The figure shows three views and two pictorial views of one solid part (mm, origin at its lowest corner). Answer the questions. A direction names the side the tool comes from. Give positions to 0.01 mm unless a question says otherwise; leave off trailing zeros. Order: outer loops, then holes, each group sorted by start corner. A loop starts at its lowest first (then second) coordinate and runs counter-clockwise, first axis right, second up. Notation, with made-up numbers: (86.25, -8.5) - (138.25, -8.5) arc R25 cw to (138.25, 13.5) - close; hole circle Ø6 at (35.25, -26). An arc over 180 degrees is marked (long way). Use a Markdown table: item, result. Add a question column.
1. A cutting plane is placed at A-A on y = 2.1. Determine the outline of the cut face in (x, z).
2. A cutting plane is placed at B-B on x = 2. Determine the outline of the cut face in (y, z), and give its area (3 significant figures).
3. For a pull along X with two mould halves and no side action, classify the marked faces 3, 4 and 5 as released by +X, released by -X, zero draft, split by the parting line, or undercut.
4. Consider L1, parallel to X at y = 6.25, z = 4.8 (3 decimals); L2, parallel to Y at x = 2.5, z = 3; L3, parallel to Y at x = 2.5, z = 5.25. Determine where each line is inside the solid, lowest interval first.
5. Which of the six approach directions +Z, -Z, +X, -X, +Y, -Y give full straight-line access (tool end or side, diameter ignored) to the marked faces 1 and 2?
6. A cutting plane is placed at D-D on y = 8.75. Determine the outline of the cut face in (x, z) (3 decimals), and give its area (3 significant figures).
7. Flat-ended cylindrical pins translate along their axes: P1, Ø0.9, axis at x = 3.5, z = 4.5, coming from the +Y side; P2, Ø1.3, axis at x = 3.5, z = 2, coming from the +Y side. Find the tip coordinate at first contact, or state that the pin passes through.
8. A cutting plane is placed at C-C on z = 6.5. Determine the outline of the cut face in (x, y).
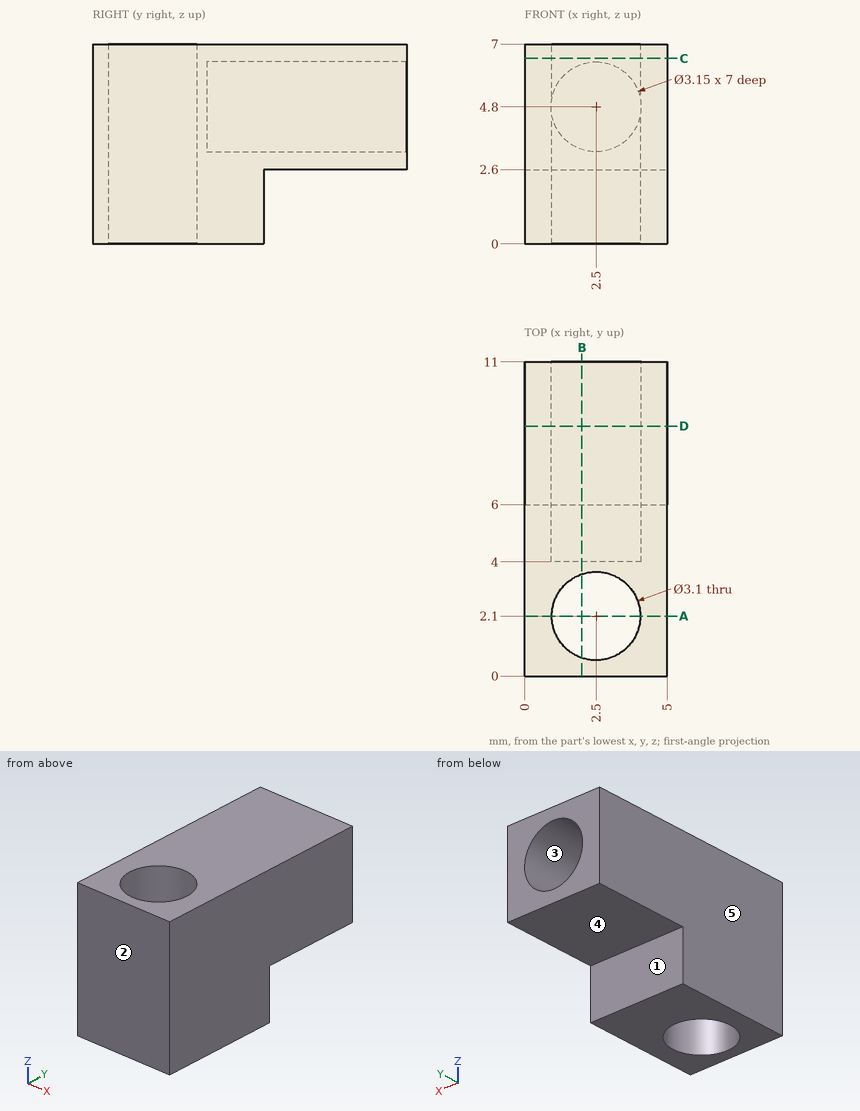
Output values:
| question | item | result |
|---|---|---|
| 1 | outline | (0, 0) - (0.95, 0) - (0.95, 7) - (0, 7) - close; (4.05, 0) - (5, 0) - (5, 7) - (4.05, 7) - close |
| 2 | outline | (0, 0) - (0.63, 0) - (0.63, 7) - (0, 7) - close; (3.57, 0) - (6, 0) - (6, 2.6) - (11, 2.6) - (11, 3.31) - (4, 3.31) - (4, 6.29) - (11, 6.29) - (11, 7) - (3.57, 7) - close |
| 2 | area | 22.6 mm² |
| 3 | face 3 | undercut |
| 3 | face 4 | zero draft |
| 3 | face 5 | released by -X |
| 4 | L1 | 0 to 0.925, 4.075 to 5 |
| 4 | L2 | 0 to 0.55, 3.65 to 11 |
| 4 | L3 | 0 to 0.55, 3.65 to 4 |
| 5 | face 1 | -Z, +X, -X, +Y |
| 5 | face 2 | +Z, -Z, +X, -X, -Y |
| 6 | outline | (0, 2.6) - (5, 2.6) - (5, 7) - (0, 7) - close; hole circle Ø3.15 at (2.5, 4.8) |
| 6 | area | 14.2 mm² |
| 7 | P1 | y = 4 |
| 7 | P2 | y = 11 |
| 8 | outline | (0, 0) - (5, 0) - (5, 11) - (0, 11) - close; hole circle Ø3.1 at (2.5, 2.1) |
